The model under review builds one solid part; all positions refer to its coordinate system, in mm. Face numbers are marked on the shaded views. A direction names the side the tool comes from. Round coordinates to 2 decimals unless told otherwise and drop trailing zeros. Loops run counter-clockwise (first coordinate to the right, second up) from the corner with the lowest first, then second, coordinate; pieces in that order, holes last. Notation, with made-up numbers: (43, 13.25) -> (54, 13.25) arc R7 ccw to (54, 21.25) -> close; hole circle Ø6 at (-5.75, -22). An arc over 180 degrees is marked (long way). Use a Markdown table: item, result. Add a question column.
1) Insertion check: pin 1 (2 mm diameter, centred on y = -77, z = 19, fed in from +X); pin 2 (4 mm diameter, centred on y = -41.5, z = 34, fed in from -X); pin 3 (12.5 mm diameter, centred on y = -74.5, z = 24, fed in from -X); pin 4 (4.5 mm diameter, centred on x = -10.48, z = 31.43, fed in from +Y). Each pin has a flat end and moves straight along its axis. Give the tip position at first contact, or say it passes through.
2) Consider section C-C on x = 20.5. Give the boundary of the cut face in (y, z), plus the area to 3 significant figures.
3) Consider section A-A on y = -74. Give the boundary of the cut face in (x, z).
4) Mouldability with a two-part tool opening along X and no side actions: class the marked faces 4, 5 and 6 as released by +X, released by -X, zero draft, split by the parting line, or undercut.
5) Wall thickness on probe 1 along Z at (x, y) = (0, -82.75); probe 2 along Y at (x, z) = (58, 25.5); probe 3 along X at (y, z) = (17, 37.5): over which ranges is each line inside the solid? List them lowest first.
6) Consider section B-B on x = 0. Give the boundary of the cut face in (y, z).
7) For the marked faces 1, 2 and 3, list the 3-axis set-ups (+Z, -Z, +X, -X, +Y, -Y) from which the entire face can be reached by the end or side of a thin tool; tool diameter is ignored.
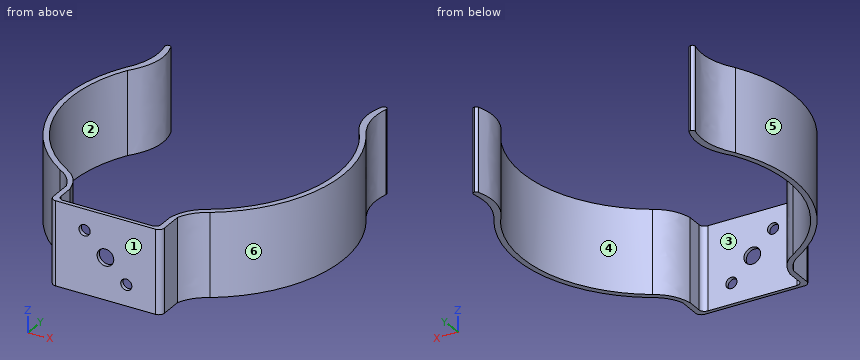
from build123d import *

# Parameters (mm, degrees)
BOSS_EXTRUDE1_DEPTH = 38.1
SKETCH2_R           = 3.81
SKETCH2_R_2         = 2.54
CUT_EXTRUDE1_DEPTH  = 2.54
FILLET1_R           = 1.27
FILLET2_R           = 2.54
SCALE1_SCALE        = 1.1


with BuildPart() as part:
    # Sketch1 → Boss-Extrude1 (new body)
    with BuildSketch(Plane.XY):
        with BuildLine():
            Line((-51.030503122, 56.023178588), (-48.490503122, 56.023178588))
            add(Edge.make_bspline(
                [(-48.490503122, 56.023178588), (-43.069252532, 42.611394773), (-53.01543557, 30.091280986)],
                knots=[0, 0, 0, 1, 1, 1], degree=2))
            ThreePointArc((-53.01543557, 30.091280986), (-59.06455096, -15.083117047), (-32.096486043, -51.826028053))
            add(Edge.make_bspline(
                [(-32.096486043, -51.826028053), (-26.666596777, -55.080730316), (-24.15411201, -59.274056829), (-22.86, -65.092330549)],
                knots=[0, 0, 0, 0, 1, 1, 1, 1], degree=3))
            Line((-22.86, -65.092330549), (-22.86, -74.449178354))
            Line((-22.86, -74.449178354), (22.86, -74.449178354))
            Line((22.86, -74.449178354), (22.86, -65.092330549))
            add(Edge.make_bspline(
                [(32.096486043, -51.826028053), (26.666596777, -55.080730316), (24.15411201, -59.274056829), (22.86, -65.092330549)],
                knots=[0, 0, 0, 0, 1, 1, 1, 1], degree=3))
            ThreePointArc((32.096486043, -51.826028053), (59.06455096, -15.083117047), (53.01543557, 30.091280986))
            add(Edge.make_bspline(
                [(48.490503122, 56.023178588), (43.069252532, 42.611394773), (53.01543557, 30.091280986)],
                knots=[0, 0, 0, 1, 1, 1], degree=2))
            Line((48.490503122, 56.023178588), (51.030503122, 56.023178588))
            add(Edge.make_bspline(
                [(55.224412052, 31.34508436), (47.144066751, 43.196956405), (51.030503122, 56.023178588)],
                knots=[0, 0, 0, 1, 1, 1], degree=2))
            ThreePointArc((55.224412052, 31.34508436), (61.651768505, -15.208860583), (34.310656711, -53.432469867))
            add(Edge.make_bspline(
                [(34.310656711, -53.432469867), (27.932475889, -56.813983763), (25.4, -63.5)],
                knots=[0, 0, 0, 1, 1, 1], degree=2))
            Line((25.4, -63.5), (25.4, -76.2))
            Line((25.4, -76.2), (-25.4, -76.2))
            Line((-25.4, -76.2), (-25.4, -63.5))
            add(Edge.make_bspline(
                [(-34.310656711, -53.432469867), (-27.932475889, -56.813983763), (-25.4, -63.5)],
                knots=[0, 0, 0, 1, 1, 1], degree=2))
            ThreePointArc((-34.310656711, -53.432469867), (-61.651768505, -15.208860583), (-55.224412052, 31.34508436))
            add(Edge.make_bspline(
                [(-55.224412052, 31.34508436), (-47.144066751, 43.196956405), (-51.030503122, 56.023178588)],
                knots=[0, 0, 0, 1, 1, 1], degree=2))
        make_face()
    extrude(amount=BOSS_EXTRUDE1_DEPTH)

    # Sketch2 → Cut-Extrude1 (cut)
    with BuildSketch(Plane(origin=(0, -74.449178354, 0), x_dir=(1, 0, 0), z_dir=(0, 1, 0))):
        with Locations((0, -19.05)):
            Circle(SKETCH2_R)
        with Locations((9.525, -9.525)):
            Circle(SKETCH2_R_2)
        with Locations((-9.525, -28.575)):
            Circle(SKETCH2_R_2)
    extrude(amount=-CUT_EXTRUDE1_DEPTH, mode=Mode.SUBTRACT)

    # Fillet1
    fillet1_edges = [part.edges().sort_by_distance(p)[0] for p in [
        (51.030503122, 56.023178588, 19.05),
        (48.490503122, 56.023178588, 19.05),
        (-48.490503122, 56.023178588, 19.05),
        (-51.030503122, 56.023178588, 19.05),
    ]]
    fillet(fillet1_edges, radius=FILLET1_R)

    # Fillet2
    fillet2_edges = [part.edges().sort_by_distance(p)[0] for p in [
        (-22.86, -74.449178354, 19.05),
        (22.86, -74.449178354, 19.05),
        (25.4, -76.2, 19.05),
        (-25.4, -76.2, 19.05),
    ]]
    fillet(fillet2_edges, radius=FILLET2_R)


with BuildPart() as part_1:
    # Scale1: scaled about (0, 0, 0)
    add(part.part.scale(SCALE1_SCALE))


solid = part_1.part
Result set:
| question | item | result |
|---|---|---|
| 1 | pin 1 | x = 27.94 |
| 1 | pin 2 | x = -57.61 |
| 1 | pin 3 | x = -28.62 |
| 1 | pin 4 | through |
| 2 | outline | (-83.82, 0) -> (-81.89, 0) -> (-81.89, 41.91) -> (-83.82, 41.91) -> close |
| 2 | area | 80.7 mm2 |
| 3 | outline | (-27.94, 0) -> (-25.15, 0) -> (-25.15, 41.91) -> (-27.94, 41.91) -> close; (25.15, 0) -> (27.94, 0) -> (27.94, 41.91) -> (25.15, 41.91) -> close |
| 4 | face 4 | undercut |
| 4 | face 5 | released by -X |
| 4 | face 6 | released by +X |
| 5 | probe 1 | 0 to 16.76, 25.15 to 41.91 |
| 5 | probe 2 | -38.92 to -33.65, 33.5 to 39.15 |
| 5 | probe 3 | -67.75 to -64.87, 64.87 to 67.75 |
| 6 | outline | (-83.82, 0) -> (-81.89, 0) -> (-81.89, 16.76) -> (-83.82, 16.76) -> close; (-83.82, 25.15) -> (-81.89, 25.15) -> (-81.89, 41.91) -> (-83.82, 41.91) -> close |
| 7 | face 1 | +Z, -Z, +X, -X, -Y |
| 7 | face 2 | +Z, -Z |
| 7 | face 3 | +Z, -Z, +Y |
